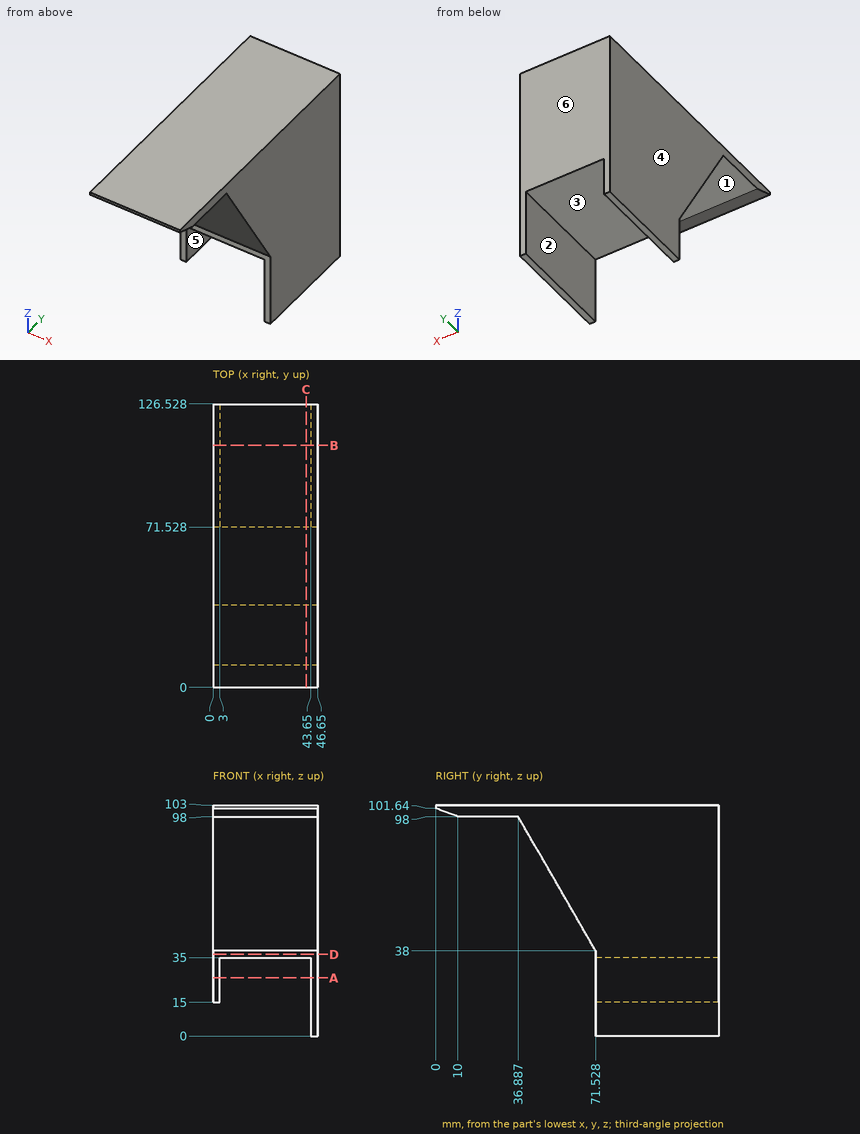
Input: dimensioned drawing with shaded views. Units: mm. Origin: part minimum x, y, z. A direction names the side the tool comes from. Coordinates: 2 decimals unless noted, no trailing zeros. Order: outer loops, then holes, each group sorted by start corner. A loop starts at its lowest first (then second) coordinate and runs counter-clockwise, first axis right, second up. Notation, with made-up numbers: (50.5, 70) - (81.5, 70) arc R26 cw to (81.5, 95) - close; hole circle Ø7 at (23, -23). An arc over 180 degrees is marked (long way). Put each result on its own line as item: value.
1. Contact query for flat-ended pins moving along their axis: pin 1 Ø13.5 at (x, y) = (15.5, 23.5) entering from -Z; pin 2 Ø6 at (x, z) = (15, 53.5) entering from -Y; pin 3 Ø8 at (x, z) = (6.5, 21.5) entering from +Y; pin 4 Ø1.5 at (x, y) = (2, 96.5) entering from -Z. Output: stop coordinate, or through.
Report:
pin 1: stops at z = 98
pin 2: stops at y = 60.85
pin 3: stops at y = 126.53
pin 4: stops at z = 15
2. Draft query along X for the marked faces 1, 2, 3 and 4. Return one class per face: pulls with the +X half, pulls with the -X half, needs draft (parallel to the pull), parting line crosses it, or undercut.
Report:
face 1: needs draft
face 2: undercut
face 3: undercut
face 4: pulls with the -X half
3. Cut plane D-D on z = 36.5. Return the cut outline in (x, y).
Report:
outline: (0, 71.53) - (46.65, 71.53) - (46.65, 126.53) - (0, 126.53) - close
4. Cut plane C-C on x = 41.5. Return the cut outline in (y, z), then the cut area to 3 significant figures.
Report:
outline: (0, 101.64) - (10, 98) - (36.89, 98) - (71.53, 38) - (71.53, 35) - (126.53, 35) - (126.53, 103) - (0, 103) - close
area: 5,120 mm2
5. Cut plane A-A on z = 26. Return the cut outline in (x, y).
Report:
outline: (0, 71.53) - (3, 71.53) - (3, 126.53) - (0, 126.53) - close; (43.65, 71.53) - (46.65, 71.53) - (46.65, 126.53) - (43.65, 126.53) - close
6. Cut plane B-B on y = 108. Return the cut outline in (x, z), then the cut area to 3 significant figures.
Report:
outline: (0, 15) - (3, 15) - (3, 35) - (43.65, 35) - (43.65, 0) - (46.65, 0) - (46.65, 103) - (0, 103) - close
area: 3,340 mm2
7. Reachability of the marked faces 5 and 6 from +Z, -Z, +X, -X, +Y, -Y: full face, straight path, thin tool, end or side. Return the list, or none.
Report:
face 5: -Z, +Y, -Y
face 6: +Z, -Z, +X, -X, +Y
8. Line query: line 1 along X through (y, z) = (112, 13); line 2 along Z through (x, y) = (9, 17); line 3 along Z through (x, y) = (43, 94). Output: solid intervals per line, ascending.
Report:
line 1: x = 43.65 to 46.65
line 2: z = 98 to 103
line 3: z = 35 to 103
